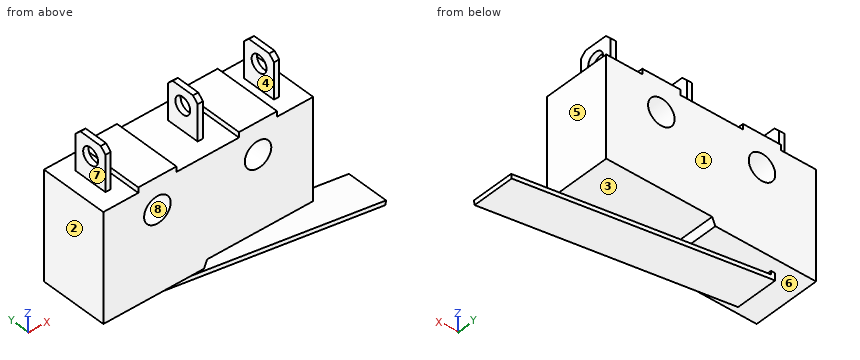
```python
from build123d import *

# Parameters (mm, degrees)
EXTRUDE_1_DEPTH                        = 6.4
SKETCH_3_R                             = 1.25
CUT_EXTRUDE_1_DEPTH                    = 13.844454056
EXTRUDE_START                          = -1.6
SKETCH_4_W                             = 3.9
SKETCH_4_H                             = 3.2
SKETCH_4_R                             = 0.8
EXTRUDE_2_DEPTH                        = 0.5
CHAMFER_1_SIZE                         = 0.5
PATTERN_LINEAR_1_COUNT                 = 2
PATTERN_LINEAR_1_PITCH                 = 8.7
CHAMFER_1_OF_PATTERN_LINEAR_1_SIZE     = 0.5
PATTERN_LINEAR_1_COL_COUNT             = 2
PATTERN_LINEAR_1_COL_PITCH             = 15.9
CHAMFER_1_OF_PATTERN_LINEAR_1_COL_SIZE = 0.5
SKETCH_6_W                             = 0.4
SKETCH_6_H                             = 4
SKETCH_7_W                             = 3.6
SKETCH_7_H                             = 6.4
EXTRUDE_4_DEPTH                        = 0.5


with BuildPart() as part:
    # Sketch 1 → Extrude 1 (new body)
    with BuildSketch(Plane(origin=(0, 0, 0), x_dir=(1, 0, 0), z_dir=(0, 1, 0))):
        Polygon((-0.4, 5.1), (-0.1, 4.4), (9.9, 4.4), (9.9, -5.1), (-9.9, -5.1), (-9.9, 5.1), align=None)
    extrude(amount=EXTRUDE_1_DEPTH)

    # Sketch 3 → Cut-Extrude 1 (cut, through all)
    with BuildSketch(Plane(origin=(0, 6.4, 0), x_dir=(1, 0, 0), z_dir=(0, 1, 0))):
        with Locations(Location((-4.8, -2.6, 0), (0, 0, 270))):
            Circle(SKETCH_3_R)
        with Locations(Location((4.7, -2.6, 0), (0, 0, 270))):
            Circle(SKETCH_3_R)
    extrude(amount=-CUT_EXTRUDE_1_DEPTH, mode=Mode.SUBTRACT)

    # Sketch 4 → Extrude 2 (add)
    with BuildSketch(Plane.ZY.offset(9.9).offset(EXTRUDE_START)):
        with Locations((7.05, 3.2)):
            Rectangle(SKETCH_4_W, SKETCH_4_H)
        with Locations((7.4, 3.2)):
            Circle(SKETCH_4_R, mode=Mode.SUBTRACT)
    extrude_2 = extrude(amount=-EXTRUDE_2_DEPTH)

    # Chamfer 1
    chamfer_1_edges = [part.edges().sort_by_distance(p)[0] for p in [
        (-8.05, 4.8, 9),
        (-8.05, 1.6, 9),
    ]]
    chamfer(chamfer_1_edges, length=CHAMFER_1_SIZE)

    # Pattern Linear 1: Extrude 2 ×2
    with Locations(*[(i * PATTERN_LINEAR_1_PITCH, 0, 0) for i in range(1, PATTERN_LINEAR_1_COUNT)]):
        add(extrude_2)

    # Chamfer 1 of Pattern Linear 1
    chamfer_1_of_pattern_linear_1_edges = [part.edges().sort_by_distance(p)[0] for p in [
        (0.65, 4.8, 9),
        (0.65, 1.6, 9),
    ]]
    chamfer(chamfer_1_of_pattern_linear_1_edges, length=CHAMFER_1_OF_PATTERN_LINEAR_1_SIZE)

    # Pattern Linear 1 col: Extrude 2 ×2
    with Locations(*[(i * PATTERN_LINEAR_1_COL_PITCH, 0, 0) for i in range(1, PATTERN_LINEAR_1_COL_COUNT)]):
        add(extrude_2)

    # Chamfer 1 of Pattern Linear 1 col
    chamfer_1_of_pattern_linear_1_col_edges = [part.edges().sort_by_distance(p)[0] for p in [
        (7.85, 4.8, 9),
        (7.85, 1.6, 9),
    ]]
    chamfer(chamfer_1_of_pattern_linear_1_col_edges, length=CHAMFER_1_OF_PATTERN_LINEAR_1_COL_SIZE)

    # Sweep 1: sweep along a path in Sketch 5
    with BuildLine(Plane(origin=(0, 3.2, 0), x_dir=(1, 0, 0), z_dir=(0, 1, 0))) as sweep_1_path:
        Line((-6.9, 5.1), (-6.9, 5.6))
        Line((-6.9, 5.6), (17.8, 9.461346915))
    # Sketch 6 → Sweep 1 (sweep)
    with BuildSketch(Plane(origin=(0, 0, -5.1), x_dir=(-1, 0, 0), z_dir=(0, 0, -1))):
        with Locations((6.9, 3.2)):
            Rectangle(SKETCH_6_W, SKETCH_6_H)
    sweep(path=sweep_1_path.line, transition=Transition.RIGHT)

    # Sketch 7 → Extrude 4 (add)
    with BuildSketch(Plane.XY.offset(5.1)):
        with Locations((-4.8, 3.2)):
            Rectangle(SKETCH_7_W, SKETCH_7_H)
        with Locations((4.7, 3.2)):
            Rectangle(SKETCH_7_W, SKETCH_7_H)
    extrude(amount=EXTRUDE_4_DEPTH)


solid = part.part
```
The listing builds one solid part. Answer for the finished solid, in the listing's coordinates (mm). Face numbers are marked on the shaded views. A direction names the side the tool comes from. Round coordinates to 2 decimals unless told otherwise and drop trailing zeros. Loops run counter-clockwise (first coordinate to the right, second up) from the corner with the lowest first, then second, coordinate; pieces in that order, holes last.
1) A cutting plane is placed at C-C on z = -4. Determine the outline of the cut face in (x, y), plus the area to 3 significant figures.
Outcome:
outline: (-9.9, 0) - (9.9, 0) - (9.9, 6.4) - (-9.9, 6.4) - close
area: 127 mm2
2) A cutting plane is placed at A-A on z = 2.6. Determine the outline of the cut face in (x, y).
Outcome:
outline: (-9.9, 0) - (-6.05, 0) - (-6.05, 6.4) - (-9.9, 6.4) - close; (-3.55, 0) - (3.45, 0) - (3.45, 6.4) - (-3.55, 6.4) - close; (5.95, 0) - (9.9, 0) - (9.9, 6.4) - (5.95, 6.4) - close
3) A cutting plane is placed at B-B on x = -4.8. Determine the outline of the cut face in (y, z).
Outcome:
outline: (0, -5.1) - (6.4, -5.1) - (6.4, 1.35) - (0, 1.35) - close; (0, 3.85) - (6.4, 3.85) - (6.4, 5.6) - (0, 5.6) - close; (1.2, -6.13) - (5.2, -6.13) - (5.2, -5.73) - (1.2, -5.73) - close
4) A cutting plane is placed at D-D on x = 15.5. Determine the outline of the cut face in (y, z).
Outcome:
outline: (1.2, -9.3) - (5.2, -9.3) - (5.2, -8.9) - (1.2, -8.9) - close
5) For the marked faces 1, 2, 3, 4 and 5, determine the directions among +Z, -Z, +X, -X, +Y, -Y from which every point of the face is accessible in a straight line to the end or side of a thin tool.
Outcome:
face 1: +Z, -Z, +X, -X, +Y
face 2: +Z, -Z, -X, +Y, -Y
face 3: +X, +Y, -Y
face 4: +Z, +Y, -Y
face 5: +Z, +X, +Y, -Y
6) Given P1, Ø2, axis at y = 3.2, z = 7.4, coming from the +X side; P2, Ø1.5, axis at x = 2.5, y = 2.5, coming from the +Z side; P3, Ø0.6, axis at x = -8, z = 7.5, coming from the +Y side, each flat-ended and moving along its own axis, determine where each tip first touches the part or whether it passes through.
Outcome:
P1: stops at x = 8.1
P2: stops at z = 5.6
P3: stops at y = 4.8
7) Consider line 1 (X direction, y = 6, z = 2.5); line 2 (Z direction, x = 5.25, y = 2); line 3 (Y direction, x = 0.65, z = 7.4). Determine where each line is inside the solid, lowest interval first.
Outcome:
line 1: x = -9.9 to -6.05, -3.55 to 3.45, 5.95 to 9.9
line 2: z = -7.7 to -7.3, -4.4 to 1.48, 3.72 to 5.6
line 3: y = 1.6 to 2.4, 4 to 4.8
8) For a pull along X with two mould halves and no side action, classify the marked faces 6, 7 and 8 as released by +X, released by -X, zero draft, split by the parting line, or undercut.
Outcome:
face 6: zero draft
face 7: released by -X
face 8: undercut
